from build123d import *

# Parameters (mm, degrees)
SKETCH1_W           = 18.5
SKETCH1_H           = 24
SKETCH1_R           = 0.625
BOSS_EXTRUDE1_DEPTH = 2
SKETCH2_W           = 16.5
SKETCH2_H           = 2.5
BOSS_EXTRUDE2_DEPTH = 2.5
SKETCH3_W           = 16.5
SKETCH3_H           = 2.5
BOSS_EXTRUDE3_DEPTH = 0.8
FILLET2_R           = 2.5


with BuildPart() as part:
    # Sketch1 → Boss-Extrude1 (new body)
    with BuildSketch(Plane(origin=(0, 0, 0), x_dir=(1, 0, 0), z_dir=(0, 1, 0))):
        Rectangle(SKETCH1_W, SKETCH1_H)
        with BuildLine():
            Line((-4.85, -12), (-9.25, -12))
            Line((-9.25, -12), (-9.25, -14.2))
            ThreePointArc((-9.25, -14.2), (-7.05, -16.4), (-4.85, -14.2))
            Line((-4.85, -14.2), (-4.85, -12))
        make_face()
        with Locations((-7.05, -14.2)):
            Circle(SKETCH1_R, mode=Mode.SUBTRACT)
        with BuildLine():
            Line((9.25, -12), (4.85, -12))
            Line((4.85, -12), (4.85, -14.2))
            ThreePointArc((4.85, -14.2), (7.05, -16.4), (9.25, -14.2))
            Line((9.25, -14.2), (9.25, -12))
        make_face()
        with Locations((7.05, -14.2)):
            Circle(SKETCH1_R, mode=Mode.SUBTRACT)
    extrude(amount=BOSS_EXTRUDE1_DEPTH)

    # Sketch2 → Boss-Extrude2 (add)
    with BuildSketch(Plane.XZ):
        with Locations((0, -10.75)):
            Rectangle(SKETCH2_W, SKETCH2_H)
    extrude(amount=BOSS_EXTRUDE2_DEPTH)

    # Sketch3 → Boss-Extrude3 (add)
    with BuildSketch(Plane(origin=(0, -2.5, 0), x_dir=(-1, 0, 0), z_dir=(0, -1, 0))):
        with Locations((0, 13.25)):
            Rectangle(SKETCH3_W, SKETCH3_H)
    extrude(amount=-BOSS_EXTRUDE3_DEPTH)

    # Fillet2
    fillet2_edges = [part.edges().sort_by_distance(p)[0] for p in [
        (-8.25, -2.1, -14.5),
        (8.25, -2.1, -14.5),
    ]]
    fillet(fillet2_edges, radius=FILLET2_R)


solid = part.part
Here's how the part is built. I have some questions about the finished solid (model axes, mm). A direction names the side the tool comes from. Give positions to 0.01 mm unless a question says otherwise; leave off trailing zeros. Order: outer loops, then holes, each group sorted by start corner. A loop starts at its lowest first (then second) coordinate and runs counter-clockwise, first axis right, second up. Notation, with made-up numbers: (70.5, 62) -> (82.5, 62) arc R6 cw to (82.5, 68) -> close; hole circle Ø2 at (61.5, 9). An arc over 180 degrees is marked (long way). Use a Markdown table: item, result. Add a question column.
Item 1: I need wall thicknesses on line 1 (X direction, y = 1.35, z = 14.2) (3 decimals); line 2 (Y direction, x = -2.5, z = 8); line 3 (Z direction, x = 7.05, y = 1.3) (3 decimals). Which ranges of each line are inside material? Lowest first, please.
Item 2: Will these pins go through, and if not, where does the flat tip stop? pin 1 (1 mm diameter, centred on x = 2, z = -3, fed in from -Y); pin 2 (2 mm diameter, centred on y = -1.5, z = -11, fed in from -X); pin 3 (1.2 mm diameter, centred on x = 0.5, y = -2, fed in from +Z).
Item 3: Imagine slicing it at B-B on x = -7.05. Please give me the cut outline in (y, z) (3 decimals), plus the area to 3 significant figures.
Item 4: For faces 5 (the face through (0, -1, -9.5)), 6 (the face through (0, -1.7, -13)), 7 (the face through (0, 1, 12)), which set-ups out of +Z, -Z, +X, -X, +Y, -Y let a thin tool reach every point of the face, with its end or its side?
Item 5: If we mould it in two halves opening along X, with no side actions, what happens to faces 1 (the face through (7.537, -2.094, -13.748)), 2 (the face through (-9.25, 1, 1)), 3 (the face through (6.589, 0.986, 13.778)), 4 (the face through (0, 0, 2))? For each: pulls with the +X half, pulls with the -X half, needs draft (parallel to the pull), parting line crosses it, or undercut.
Item 6: Imagine slicing it at A-A on z = -10.5. Please give me the cut outline in (x, y).
Item 7: Imagine slicing it at C-C on x = 1.5. Please give me the cut outline in (y, z), plus the area to 4 significant figures.
Item 8: Imagine slicing it at D-D on y = -0.7. Please give me the cut outline in (x, z), plus the area to 4 significant figures.
Data:
| question | item | result |
|---|---|---|
| 1 | line 1 | x = -9.25 to -7.675, -6.425 to -4.85, 4.85 to 6.425, 7.675 to 9.25 |
| 1 | line 2 | y = 0 to 2 |
| 1 | line 3 | z = -12 to 13.575, 14.825 to 16.4 |
| 2 | pin 1 | stops at y = 0 |
| 2 | pin 2 | stops at x = -8.25 |
| 2 | pin 3 | stops at z = -9.5 |
| 3 | outline | (-2.5, -14.135) -> (-1.7, -14.135) -> (-1.7, -12) -> (2, -12) -> (2, 13.575) -> (0, 13.575) -> (0, -9.5) -> (-2.5, -9.5) -> close; (0, 14.825) -> (2, 14.825) -> (2, 16.4) -> (0, 16.4) -> close |
| 3 | area | 62.3 mm² |
| 4 | face 5 | +Z, +X, -X, -Y |
| 4 | face 6 | -Z, +X, -X, +Y |
| 4 | face 7 | +Z, +Y, -Y |
| 5 | face 1 | pulls with the +X half |
| 5 | face 2 | pulls with the -X half |
| 5 | face 3 | undercut |
| 5 | face 4 | needs draft |
| 6 | outline | (-9.25, 0) -> (-8.25, 0) -> (-8.25, -2.5) -> (8.25, -2.5) -> (8.25, 0) -> (9.25, 0) -> (9.25, 2) -> (-9.25, 2) -> close |
| 7 | outline | (-2.5, -14.5) -> (-1.7, -14.5) -> (-1.7, -12) -> (2, -12) -> (2, 12) -> (0, 12) -> (0, -9.5) -> (-2.5, -9.5) -> close |
| 7 | area | 56.25 mm² |
| 8 | outline | (-8.25, -12) -> (8.25, -12) -> (8.25, -9.5) -> (-8.25, -9.5) -> close |
| 8 | area | 41.25 mm² |
